```python
from build123d import *

# Parameters (mm, degrees)
SKETCH1_W           = 90
SKETCH1_H           = 20
SKETCH1_R           = 1.75
SKETCH1_R_2         = 3
BOSS_EXTRUDE1_DEPTH = 10
CHAMFER1_SIZE       = 5


with BuildPart() as part:
    # Sketch1 → Boss-Extrude1 (new body)
    with BuildSketch(Plane(origin=(0, 0, 0), x_dir=(1, 0, 0), z_dir=(0, 1, 0))):
        with Locations((35, 0)):
            Rectangle(SKETCH1_W, SKETCH1_H)
        with Locations(Location((0, 0, 0), (0, 0, 270))):
            Circle(SKETCH1_R, mode=Mode.SUBTRACT)
        with Locations(Location((70, 0, 0), (0, 0, 270))):
            Circle(SKETCH1_R, mode=Mode.SUBTRACT)
        with Locations(Location((15, 0, 0), (0, 0, 270))):
            Circle(SKETCH1_R_2, mode=Mode.SUBTRACT)
        with Locations(Location((45, 0, 0), (0, 0, 270))):
            Circle(SKETCH1_R_2, mode=Mode.SUBTRACT)
    extrude(amount=BOSS_EXTRUDE1_DEPTH)

    # Chamfer1
    chamfer1_edges = [part.edges().sort_by_distance(p)[0] for p in [
        (-10, 5, -10),
        (80, 5, -10),
        (80, 5, 10),
        (-10, 5, 10),
    ]]
    chamfer(chamfer1_edges, length=CHAMFER1_SIZE)


solid = part.part
```
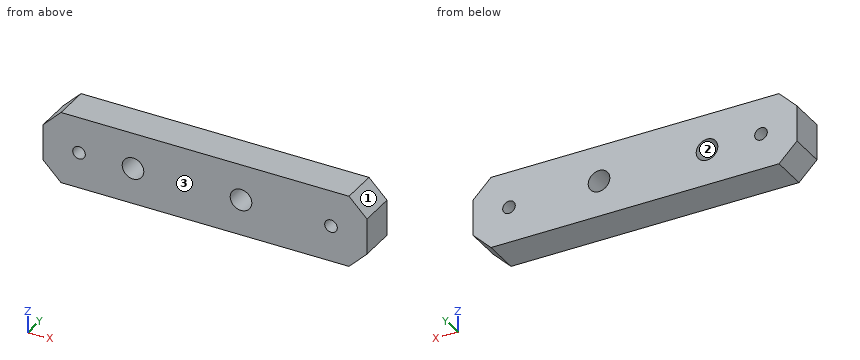
The model under review builds one solid part; all positions refer to its coordinate system, in mm. Face numbers are marked on the shaded views. Round coordinates to 2 decimals unless told otherwise and drop trailing zeros. Loops run counter-clockwise (first coordinate to the right, second up) from the corner with the lowest first, then second, coordinate; pieces in that order, holes last. Notation, with made-up numbers: M 13.5,77.5 L 41.5,77.5 A24 cw 41.5,89.5 Z; hole C 66,55.25 d3. An arc over 180 degrees is marked long. Write item = value, one per line.
Item 1: Insertion check: P1, Ø3, axis at x = 0, z = 0, coming from the +Y side. The pin has a flat end and moves straight along its axis. Give the tip position at first contact, or say it passes through.
Return value:
P1 = through
Item 2: Take a section at B-B on z = 0. Write out the cut boundary in (x, y), then the cut area to 3 significant figures.
Return value:
outline = M -10,0 L -1.75,0 L -1.75,10 L -10,10 Z; M 1.75,0 L 12,0 L 12,10 L 1.75,10 Z; M 18,0 L 42,0 L 42,10 L 18,10 Z; M 48,0 L 68.25,0 L 68.25,10 L 48,10 Z; M 71.75,0 L 80,0 L 80,10 L 71.75,10 Z
area = 710 mm2
Item 3: Take a section at A-A on x = 70. Write out the cut boundary in (y, z), then the cut area to 3 significant figures.
Return value:
outline = M 0,-10 L 10,-10 L 10,-1.75 L 0,-1.75 Z; M 0,1.75 L 10,1.75 L 10,10 L 0,10 Z
area = 165 mm2
Item 4: The part is to be moulded in two halves that separate along X. For the marked faces 1, 2 and 3, say which applies: released by +X, released by -X, zero draft, split by the parting line, or undercut.
Return value:
face_1 = released by +X
face_2 = undercut
face_3 = zero draft
Item 5: Take a section at C-C on y = 7. Write out the cut boundary in (x, z), then the cut area to 3 significant figures.
Return value:
outline = M -10,-5 L -5,-10 L 75,-10 L 80,-5 L 80,5 L 75,10 L -5,10 L -10,5 Z; hole C 0,0 d3.5; hole C 15,0 d6; hole C 45,0 d6; hole C 70,0 d3.5
area = 1,670 mm2
Item 6: Take a section at D-D on x = 45. Write out the cut boundary in (y, z).
Return value:
outline = M 0,-10 L 10,-10 L 10,-3 L 0,-3 Z; M 0,3 L 10,3 L 10,10 L 0,10 Z
Item 7: For line 1 (X direction, y = 4, z = 0); line 2 (Z direction, x = 70, y = 6); line 3 (X direction, y = 3, z = -1), list the stretches that pass through material, from the lowest coordinate up. Write a range as [from, to].
Return value:
line_1 = [-10, -1.75], [1.75, 12], [18, 42], [48, 68.25], [71.75, 80]
line_2 = [-10, -1.75], [1.75, 10]
line_3 = [-10, -1.44], [1.44, 12.17], [17.83, 42.17], [47.83, 68.56], [71.44, 80]
